Design review of the part built by this model. Coordinates are the model's own, in mm. A direction names the side the tool comes from. Give positions to 0.01 mm unless a question says otherwise; leave off trailing zeros. Order: outer loops, then holes, each group sorted by start corner. A loop starts at its lowest first (then second) coordinate and runs counter-clockwise, first axis right, second up. Notation, with made-up numbers: (-9.5, -38.75) -> (4.5, -38.75) arc R12 ccw to (4.5, -28.75) -> close; hole circle Ø10 at (57.25, 73). An arc over 180 degrees is marked (long way). Return JSON: item names as keys, results as strings.
```python
from build123d import *

# Parameters (mm, degrees)
SKETCH1_R           = 1.47
BOSS_EXTRUDE1_DEPTH = 1.5875


with BuildPart() as part:
    # Sketch1 → Boss-Extrude1 (new body, symmetric)
    with BuildSketch(Plane.XY):
        Polygon((-12.5, 35), (-50, 35), (-50, 12.5), (-53.175, 12.5), (-53.175, -12.5), (-50, -12.5), (-50, -35), (-12.5, -35), (-12.5, -31.825), (-1.47, -31.825), (-1.47, -28.125), (-3.25, -28.125), (-3.25, -25.525), (-1.47, -25.525), (-1.47, -21.825), (1.47, -21.825), (1.47, -25.525), (3.25, -25.525), (3.25, -28.125), (1.47, -28.125), (1.47, -31.825), (12.5, -31.825), (12.5, -35), (50, -35), (50, -12.5), (53.175, -12.5), (53.175, 12.5), (50, 12.5), (50, 35), (12.5, 35), (12.5, 31.825), (1.47, 31.825), (1.47, 28.125), (3.25, 28.125), (3.25, 25.525), (1.47, 25.525), (1.47, 21.825), (-1.47, 21.825), (-1.47, 25.525), (-3.25, 25.525), (-3.25, 28.125), (-1.47, 28.125), (-1.47, 31.825), (-12.5, 31.825), align=None)
        with Locations((-51.5875, 0)):
            Circle(SKETCH1_R, mode=Mode.SUBTRACT)
        with Locations((51.5875, 0)):
            Circle(SKETCH1_R, mode=Mode.SUBTRACT)
    extrude(amount=BOSS_EXTRUDE1_DEPTH, both=True)


solid = part.part
```
Item 1: Add section D-D (x = 9.5). Give the boundary of the cut face in (y, z) (1 decimal).
Result set:
{"outline": "(-31.8, -1.6) -> (31.8, -1.6) -> (31.8, 1.6) -> (-31.8, 1.6) -> close"}
Item 2: Machinability: for faces 1 (the face through (0, 21.825, 0)), 2 (the face through (-12.5, -33, 0)), 3 (the face through (-52, 12.5, 0)), which of the approach directions +Z, -Z, +X, -X, +Y, -Y give a long, thin tool a straight path to every point of the face, cutting with its end or side? Answer none if there is none.
Result set:
{"face 1": "+Z, -Z, +Y", "face 2": "+Z, -Z, -Y", "face 3": "+Z, -Z, -X, +Y"}
Item 3: For pin 1 (1.6 mm diameter, centred on y = 24, z = 1, fed in from -X); pin 2 (1 mm diameter, centred on x = 51.5, z = 0, fed in from -Y); pin 3 (1 mm diameter, centred on x = -6.5, z = -0.5, fed in from -Y) (3 decimals), all flat-tipped, find the tip position at first contact; note any pin that passes through.
Result set:
{"pin 1": "stops at x = -50", "pin 2": "stops at y = -12.5", "pin 3": "stops at y = -31.825"}
Item 4: Add section A-A (y = 0). Give the number of separate pieces and of enclosed holes in the cut face, plus the area to 3 significant figures.
Result set:
{"separate pieces": "3", "enclosed holes": "0", "area": "319 mm^2"}
Item 5: Mouldability with a two-part tool opening along Y and no side actions: class faces 4 (the face through (7, -31.825, 0)), 5 (the face through (3.25, 27, 0)), 6 (the face through (-1, 0, -1.588)) as released by +Y, released by -Y, zero draft, split by the parting line, or undercut.
Result set:
{"face 4": "released by -Y", "face 5": "undercut", "face 6": "zero draft"}
Item 6: Wall thickness on L1, parallel to Y at x = -2, z = -0.55 (3 decimals); L2, parallel to X at y = -24, z = 0; L3, parallel to Y at x = 9.5, z = -1.1 (3 decimals): over which ranges is each line inside the solid? List them lowest first. Write a range as [from, to].
Result set:
{"L1": "y = [-31.825, -28.125], [-25.525, 25.525], [28.125, 31.825]", "L2": "x = [-50, -1.47], [1.47, 50]", "L3": "y = [-31.825, 31.825]"}
Item 7: Add section B-B (y = 23). Give the boundary of the cut face in (x, z).
Result set:
{"outline": "(-50, -1.59) -> (-1.47, -1.59) -> (-1.47, 1.59) -> (-50, 1.59) -> close; (1.47, -1.59) -> (50, -1.59) -> (50, 1.59) -> (1.47, 1.59) -> close"}
